```python
from build123d import *

# Parameters (mm, degrees)
F0_W      = 205
F0_H      = 106
F1_DEPTH  = 5
F2_R      = 4.25
F3_DEPTH  = 500
F4_W      = 20
F4_H      = 10
F5_DEPTH  = 500
F6_W      = 12
F6_H      = 8
F7_DEPTH  = 500
F8_R      = 4.99999
F9_W      = 47
F9_H      = 10
F10_DEPTH = 500


# Not quite as in the source:
# - a fillet or chamfer is up to 0.001 mm smaller than in the source, because OpenCascade refuses the exact size


with BuildPart() as f1:
    # F0 (on Top) → F1 (new body)
    with BuildSketch(Plane.XY):
        with Locations((-719.1119938903, -475.8524597138)):
            Rectangle(F0_W, F0_H)
    extrude(amount=F1_DEPTH)

    # F2 (on face) → F3 (cut)
    with BuildSketch(Plane.XY.offset(5)):
        with Locations((-649.6119938903, -517.8524597138)):
            Circle(F2_R)
    extrude(amount=-F3_DEPTH, mode=Mode.SUBTRACT)

    # F4 (on face) → F5 (cut)
    with BuildSketch(Plane.XY.offset(5)):
        with Locations((-670.6119938903, -515.8524597138)):
            Rectangle(F4_W, F4_H)
    extrude(amount=-F5_DEPTH, mode=Mode.SUBTRACT)

    # F6 (on face) → F7 (cut)
    with BuildSketch(Plane.XY.offset(5)):
        with Locations((-695.1119938903, -517.8524597138)):
            Rectangle(F6_W, F6_H)
    extrude(amount=-F7_DEPTH, mode=Mode.SUBTRACT)

    # F8 (radius 5 in the source; OpenCascade refuses exactly that, so slightly less here)
    f8_edges = [f1.edges().sort_by_distance(p)[0] for p in [
        (-821.611994, -475.85246, 5),
        (-719.111994, -528.85246, 5),
        (-616.611994, -475.85246, 5),
        (-719.111994, -422.85246, 5),
    ]]
    fillet(f8_edges, radius=F8_R)

    # F9 (on face) → F10 (cut)
    with BuildSketch(Plane.XY.offset(5)):
        with Locations((-732.1119938903, -518.8524597138)):
            Rectangle(F9_W, F9_H)
    extrude(amount=-F10_DEPTH, mode=Mode.SUBTRACT)


solid = f1.part
```
Here's how the part is built. I have some questions about the finished solid (model axes, mm). A direction names the side the tool comes from. Round coordinates to 2 decimals unless told otherwise and drop trailing zeros. Order: outer loops, then holes, each group sorted by start corner. A loop starts at its lowest first (then second) coordinate and runs counter-clockwise, first axis right, second up. Notation, with made-up numbers: (8.5, 2.5) -> (20.5, 2.5) arc R19 ccw to (20.5, 38.5) -> close; hole circle Ø10 at (6, 89). An arc over 180 degrees is marked (long way). Use a Markdown table: item, result. Add a question column.
(1) For pin 1 Ø1.5 at (y, z) = (-518.5, 2.5) entering from -X; pin 2 Ø3 at (y, z) = (-483, 4) entering from +X; pin 3 Ø1.5 at (x, z) = (-740.5, 3) entering from +Y; pin 4 Ø3 at (x, y) = (-787.5, -514) entering from -Z, each with a flat end and sliding along its axis, tell me the tip position at first contact or that it passes through.
(2) Suppose I cut it at B-B, the plane z = 2.4. Please give me the cut outline in (x, y), and give its area (3 significant figures).
(3) If we mould it in two halves opening along X, with no side actions, what happens to faces 3 (the face through (-820.186, -475.11, 3.496)), 4 (the face through (-618.116, -475.11, 3.574)), 5 (the face through (-755.612, -519, 3)), 6 (the face through (-720, -475, 5))? For each: released by +X, released by -X, zero draft, split by the parting line, or undercut.
(4) For faces 1 (the face through (-660.612, -516, 3)), 2 (the face through (-717.68, -424.28, 3.5)), which set-ups out of +Z, -Z, +X, -X, +Y, -Y let a thin tool reach every point of the face, with its end or its side?
(5) I need wall thicknesses on line 1 along X through (y, z) = (-516.5, 1.3); line 2 along X through (y, z) = (-515, 1.1); line 3 along X through (y, z) = (-496, 0.5). Which ranges of each line are inside material? Lowest first, please.
Verdict:
| question | item | result |
|---|---|---|
| 1 | pin 1 | x = -821.3 |
| 1 | pin 2 | x = -617.28 |
| 1 | pin 3 | y = -423.39 |
| 1 | pin 4 | z = 0 |
| 2 | outline | (-821, -528.24) -> (-617.23, -528.24) -> (-617.23, -423.47) -> (-821, -423.47) -> close; hole (-755.61, -523.85) -> (-708.61, -523.85) -> (-708.61, -513.85) -> (-755.61, -513.85) -> close; hole (-701.11, -521.85) -> (-689.11, -521.85) -> (-689.11, -513.85) -> (-701.11, -513.85) -> close; hole (-680.61, -520.85) -> (-660.61, -520.85) -> (-660.61, -510.85) -> (-680.61, -510.85) -> close; hole circle Ø8.5 at (-649.61, -517.85) |
| 2 | area | 20,500 mm2 |
| 3 | face 3 | released by -X |
| 3 | face 4 | released by +X |
| 3 | face 5 | undercut |
| 3 | face 6 | zero draft |
| 4 | face 1 | +Z, -Z |
| 4 | face 2 | +Z, +X, -X, +Y |
| 5 | line 1 | -821.44 to -755.61, -708.61 to -701.11, -689.11 to -680.61, -660.61 to -653.64, -645.58 to -616.78 |
| 5 | line 2 | -821.49 to -755.61, -708.61 to -701.11, -689.11 to -680.61, -660.61 to -652.76, -646.46 to -616.73 |
| 5 | line 3 | -821.59 to -616.64 |
